Design review of the part built by this model. Coordinates are the model's own, in mm. A direction names the side the tool comes from. Give positions to 0.01 mm unless a question says otherwise; leave off trailing zeros. Write each loop counter-clockwise with the first axis right and the second up, starting at its lowest first coordinate (ties: lowest second). Pieces come first, ordered by that corner, then holes. Notation, with made-up numbers: (72, 21) -> (80, 21) arc R32 ccw to (80, 50) -> close; hole circle Ø2 at (-2.5, -24.5). An arc over 180 degrees is marked (long way). Put each result on its own line as item: value. Start each with the question number.
from build123d import *

# Parameters (mm, degrees)
BOSS_EXTRUDE1_DEPTH = 4
HOLE1_D             = 6
HOLE1_DEPTH         = 53
HOLE1_CBORE_D       = 16.8
HOLE1_CBORE_DEPTH   = 24
FILLET1_R           = 0.1
SCALE1_SCALE        = 0.92


with BuildPart() as part:
    # Sketch1 → Boss-Extrude1 (new body)
    with BuildSketch(Plane(origin=(2, 0, 0), x_dir=(0, 0, -1), z_dir=(1, 0, 0))):
        Polygon((11.547005384, 0), (5.773502692, 10), (-5.773502692, 10), (-11.547005384, 0), (-5.773502692, -10), (5.773502692, -10), align=None)
    extrude(amount=-BOSS_EXTRUDE1_DEPTH)

    # Sketch2 → Revolve1 (revolve)
    with BuildSketch(Plane.XY):
        Polygon((-26, 9.45), (-26, 0), (-2, 0), (-2, 9.65), (-4, 9.65), (-9, 9), (-9, 9.65), (-10, 9.65), (-15, 9), (-15, 9.65), (-16, 9.65), (-21, 9), (-21, 9.65), (-24, 9.65), align=None)
    revolve(axis=Axis((-26, 0, 0), (1, 0, 0)))

    # Sketch3 → Revolve2 (revolve)
    with BuildSketch(Plane.XY):
        Polygon((2, 6.477), (2, 0), (27, 0), (27, 6.35), (25, 6.5), (22, 6.5), (22, 6.15), (18, 6.5), (16, 6.5), (16, 6.15), (12, 6.5), (10, 6.5), (10, 5.977), (6.5, 6.327), align=None)
    revolve(axis=Axis((2, 0, 0), (1, 0, 0)))

    # Hole1
    with Locations(Plane.ZY.offset(26)):
        with Locations((0, 0)):
            CounterBoreHole(HOLE1_D / 2, HOLE1_CBORE_D / 2, HOLE1_CBORE_DEPTH, depth=HOLE1_DEPTH)

    # Fillet1
    fillet1_edges = [part.edges().sort_by_distance(p)[0] for p in [
        (-26, -9.45, 0),
        (27, -6.35, 0),
        (-26, 0, -8.4),
        (27, 0, 3),
    ]]
    fillet(fillet1_edges, radius=FILLET1_R)


with BuildPart() as part_1:
    # Scale1: scaled about (3.211544185, 0, 0)
    add(part.part.scale(SCALE1_SCALE).moved(Location((0.256923535, 0, 0))))


solid = part_1.part
Q1. Take a section at A-A on x = -11.5. Give the boundary of the cut face in (y, z).
Q2. Take a section at B-B on x = 8.5. Give the boundary of the cut face in (y, z).
Q3. Machinability: for faces 5 (the face through (25.097, 3, -1)), 6 (the face through (-19.063, -8, 3)), 7 (the face through (21.858, 2.759, -5.305)), 8 (the face through (-8.49, -1.925, -8.667)), which of the approach directions +Z, -Z, +X, -X, +Y, -Y give a long, thin tool a straight path to every point of the face, cutting with its end or side? Answer none if there is none.
Q4. Mouldability with a two-part tool opening along Y and no side actions: class faces 1 (the face through (4.138, -4.675, -3.584)), 2 (the face through (2.097, 4, -5)), 3 (the face through (-12.731, -7.544, -1.675)), 4 (the face through (0.28, 4.54, -8)) as +Y half, -Y half, draft (parallel to the pull), parting line (faces both ways), or undercut.
Q5. For pin 1 (4 mm diameter, centred on x = -14.5, z = -3.5, fed in from -Y); pin 2 (6 mm diameter, centred on x = -6.5, z = 5, fed in from -Y); pin 3 (2 mm diameter, centred on x = -15, z = 6, fed in from -Y); pin 4 (8 mm diameter, centred on x = -3.5, y = -3, fed in from -Z), all flat-tipped, find the tip position at first contact; note any pin that passes through.
Q6. To check wall thickness, follow probe 1 along X at (y, z) = (3, 6.25); probe 2 along Y at (x, z) = (-15.75, 0); probe 3 along Y at (x, z) = (-19, 0). State the ranges of each line that lie inside material, in increasing order. Write a range as from..to.
Result:
1. outline: circle Ø17.09 at (0, 0); hole circle Ø15.46 at (0, 0)
2. outline: circle Ø11.19 at (0, 0); hole circle Ø5.52 at (0, 0)
3. face 5: +Z, -Z, +X, +Y, -Y
3. face 6: none
3. face 7: +X
3. face 8: -X
4. face 1: parting line
4. face 2: draft
4. face 3: undercut
4. face 4: +Y half
5. pin 1: stops at y = -8.75
5. pin 2: stops at y = -8.54
5. pin 3: stops at y = -7.27
5. pin 4: stops at z = -10.62
6. probe 1: x = -1.58..2.1
6. probe 2: y = -8.71..-7.73, 7.73..8.71
6. probe 3: y = -8.29..-7.73, 7.73..8.29
